Here's how the part is built. I have some questions about the finished solid (model axes, mm). A direction names the side the tool comes from. Give positions to 0.01 mm unless a question says otherwise; leave off trailing zeros. Order: outer loops, then holes, each group sorted by start corner. A loop starts at its lowest first (then second) coordinate and runs counter-clockwise, first axis right, second up.
Autodesk Inventor part; units mm, degrees
ref_plane "YZ Plane" through (0, 0, 0) normal (1, 0, 0) x (0, 1, 0)
ref_plane "XZ Plane" through (0, 0, 0) normal (0, 1, 0) x (-1, 0, 0)
ref_plane "XY Plane" through (0, 0, 0) normal (0, 0, 1) x (1, 0, 0)
sketch "스케치1" plane through (0, 0, 0) normal (0, 0, 1) x (1, 0, 0)
  line L0 (-17.5, 17.5) -> (17.5, 17.5)
  line L1 (17.5, 17.5) -> (17.5, -17.5)
  line L2 (17.5, -17.5) -> (-17.5, -17.5)
  line L3 (-17.5, -17.5) -> (-17.5, 17.5)
  line L4 (-17.5, 17.5) -> (17.5, -17.5) construction
  line L5 (17.5, 17.5) -> (-17.5, -17.5) construction
  point P0 (0, 0)
  dimension "d0" = 35
  dimension "d1" = 35
extrude "돌출1" add sketch "스케치1" along normal blind 255
sketch "스케치2" plane through (0, 0, 255) normal (0, 0, 1) x (1, 0, 0)
  line L0 (-25, -25) -> (25, -25)
  line L1 (25, -25) -> (25, 25)
  line L2 (25, 25) -> (-25, 25)
  line L3 (-25, 25) -> (-25, -25)
  line L4 (-25, -25) -> (25, 25) construction
  line L5 (25, -25) -> (-25, 25) construction
  circle A0 centre (25, 25) radius 3.1
  circle A1 centre (-25, 25) radius 3.1
  circle A2 centre (-25, -25) radius 3.1
  circle A3 centre (25, -25) radius 3.1
  line L6 (-31, -31) -> (31, -31)
  line L7 (31, -31) -> (31, 31)
  line L8 (31, 31) -> (-31, 31)
  line L9 (-31, 31) -> (-31, -31)
  line L10 (-31, -31) -> (31, 31) construction
  line L11 (31, -31) -> (-31, 31) construction
  point P0 (0, 0)
  dimension "d4" = 50
  dimension "d5" = 50
  dimension "d6" = 6.2
  dimension "d9" = 360
  dimension "d11" = 62
  dimension "d12" = 62
extrude "돌출2" add sketch "스케치2" along normal blind 5 contours A2 L3 A1 L2 A0 L1 A3 L0 | L9 L8 L7 L6
sketch "스케치3" plane through (0, 0, 0) normal (0, 0, -1) x (-1, 0, 0)
  line L0 (-31, -31) -> (31, -31)
  line L1 (31, -31) -> (31, 31)
  line L2 (31, 31) -> (-31, 31)
  line L3 (-31, 31) -> (-31, -31)
  line L4 (-31, -31) -> (31, 31) construction
  line L5 (31, -31) -> (-31, 31) construction
  circle A0 centre (25, 25) radius 3.1
  circle A1 centre (25, 25) radius 3.1
  circle A2 centre (-25, 25) radius 3.1
  circle A3 centre (-25, -25) radius 3.1
  circle A4 centre (25, -25) radius 3.1
  point P0 (0, 0)
  dimension "d17" = 360
extrude "돌출3" add sketch "스케치3" along normal blind 5
fillet "모깎기1" radius 5 12 edges at (17.5, 17.5, 127.5) (17.5, -17.5, 127.5) (-17.5, 17.5, 127.5) (31, 31, -2.5) (31, -31, -2.5) (-17.5, -17.5, 127.5) (-31, -31, -2.5) (-31, 31, -2.5) (-31, -31, 257.5) (-31, 31, 257.5) (31, -31, 257.5) (31, 31, 257.5)
properties part number "post"
Q1. I'm going to push flat-ended pins straight in: P1, Ø12.5, axis at x = -5.5, z = 126.5, coming from the -Y side; P2, Ø7.5, axis at x = 0, z = 95, coming from the +Y side; P3, Ø1.5, axis at y = 6, z = 217, coming from the +X side; P4, Ø5, axis at x = -25, y = 25, coming from the -Z side. Where does each tip first touch, or does it pass through?
Filled sheet:
P1: stops at y = -17.5
P2: stops at y = 17.5
P3: stops at x = 17.5
P4: passes through
Q2. For faces 4 (the face through (-16, 16.07, 129.28)), 5 (the face through (-17.5, 0, 126)), 6 (the face through (16, -16.07, 129.28)), which set-ups out of +Z, -Z, +X, -X, +Y, -Y let a thin tool reach every point of the face, with its end or its side?
Filled sheet:
face 4: -X, +Y
face 5: -X, +Y, -Y
face 6: +X, -Y
Q3. If we section it at B-B on z = 63: List the corners of the cut face in (x, y) for me, plus the area to 3 significant figures.
Filled sheet:
outline: (-17.5, -12.5) arc R5 ccw to (-12.5, -17.5) - (12.5, -17.5) arc R5 ccw to (17.5, -12.5) - (17.5, 12.5) arc R5 ccw to (12.5, 17.5) - (-12.5, 17.5) arc R5 ccw to (-17.5, 12.5) - close
area: 1,200 mm2
Q4. If we section it at A-A on x = -1: List the corners of the cut face in (y, z) for me.
Filled sheet:
outline: (-31, -5) - (31, -5) - (31, 0) - (17.5, 0) - (17.5, 255) - (31, 255) - (31, 260) - (-31, 260) - (-31, 255) - (-17.5, 255) - (-17.5, 0) - (-31, 0) - close
Q5. Thinking about a two-plate mould opening in Y: for faces 1 (the face through (-22.54, 26.886, -2.465)), 2 (the face through (0, 31, -2)), 3 (the face through (0, -31, 257)), which applies, released by +Y, released by -Y, zero draft, split by the parting line, or undercut?
Filled sheet:
face 1: undercut
face 2: released by +Y
face 3: released by -Y
Q6. I need wall thicknesses on L1, parallel to X at y = 25, z = 258.55; L2, parallel to Z at x = -8.5, y = -23. Which ranges of each line are inside material? Lowest first, please.
Filled sheet:
L1: x = -31 to -28.1, -21.9 to 21.9, 28.1 to 31
L2: z = -5 to 0, 255 to 260
